Work out the finished part from the listing and answer in its coordinate system (mm). A direction names the side the tool comes from. Give positions to 0.01 mm unless a question says otherwise; leave off trailing zeros. Write each loop counter-clockwise with the first axis right and the second up, starting at its lowest first coordinate (ties: lowest second). Pieces come first, ordered by that corner, then holes.
1) Straight lines are drawn through the part: probe 1 along Y at (x, z) = (-7.55, 10); probe 2 along X at (y, z) = (3, 10.5); probe 3 along Y at (x, z) = (7, 10.5). For each, find the intervals that lie inside material, in ascending order.
2) Find section B-B (x = 0). Determine the outline of the cut face in (y, z) (3 decimals), plus the area to 3 significant figures.
3) Find section D-D (z = 6.75). Determine the outline of the cut face in (x, y).
4) Determine the mould class of faces 1 (the face through (7, 0, 0)), 2 (the face through (31, 9.76, 2.46)), 3 (the face through (25.543, -13.498, 2.524)) for opening direction X: pulls with the +X half, pulls with the -X half, needs draft (parallel to the pull), parting line crosses it, or undercut.
5) Find section A-A (z = 13). Determine the outline of the cut face in (x, y), plus the area to 3 significant figures.
6) A tool of negligible diameter and unlimited length cuts with its end or side. For faces 4 (the face through (10.503, 0, 11)), 5 (the face through (8, 10, 11)), 6 (the face through (-8, -6.2, 11.6)), 7 (the face through (8, -10, 11)), 8 (the face through (-11.26, 0.18, 5.71)), from which of +Z, -Z, +X, -X, +Y, -Y can it reach the whole face along a straight path? Write none if from no direction.
7) Given pin 1 Ø1.5 at (x, z) = (9, 10.5) entering from +Y; pin 2 Ø3 at (y, z) = (-1.5, 11) entering from +X; pin 3 Ø2.5 at (x, z) = (-8, 11) entering from -Y, each flat-ended and moving along its own axis, determine where each tip first touches the part or whether it passes through.
8) Find section C-C (y = -5). Determine the outline of the cut face in (x, z).
```python
from build123d import *

# Parameters (mm, degrees)
SKETCH_1_R                     = 32.5
EXTRUDE_1_DEPTH                = 5
PATTERN_CIRCULAR_1_COUNT       = 3
SKETCH_5_W                     = 5
SKETCH_5_H                     = 20
EXTRUDE_2_DEPTH                = 10
HOLE_WIZARD_M3_1_2_D           = 3.4
HOLE_WIZARD_M3_1_2_CBORE_D     = 6.5
HOLE_WIZARD_M3_1_2_CBORE_DEPTH = 3.4
F_4_0MM_1_D                    = 4
FILLET_1_R                     = 2.5
FILLET_2_R                     = 2.5


with BuildPart() as part:
    # 스케치1 → 보스-돌출1 (new body)
    with BuildSketch(Plane.XY):
        Circle(SKETCH_1_R)
    extrude(amount=EXTRUDE_1_DEPTH)

    # 스케치4 → Hole Wizard M3 _ _1 (revolve, cut)
    with BuildSketch(Plane(origin=(0, 27.5, 5), x_dir=(0, -1, 0), z_dir=(1, 0, 0))):
        Polygon((0, 0), (0, 6.021463052), (1.7, 5), (1.7, 0.020977491), (1.725, 0), align=None)
    hole_wizard_m3_1 = revolve(axis=Axis((0, 27.5, 11.35), (0, 0, -1)), mode=Mode.SUBTRACT)

    # 원형 패턴1: Hole Wizard M3 _ _1 ×3 about axis
    pattern_circular_1_axis = Axis((0, -0.077690761, 0), (0, 0, 1))
    for i in range(1, PATTERN_CIRCULAR_1_COUNT):
        add(hole_wizard_m3_1.rotate(pattern_circular_1_axis, i * 360 / PATTERN_CIRCULAR_1_COUNT), mode=Mode.SUBTRACT)

    # 스케치5 → 보스-돌출2 (add)
    with BuildSketch(Plane.XY.offset(5)):
        with Locations((-8.003327874, 0)):
            Rectangle(SKETCH_5_W, SKETCH_5_H)
        with Locations((8.003327874, 0)):
            Rectangle(SKETCH_5_W, SKETCH_5_H)
    extrude(amount=EXTRUDE_2_DEPTH)

    # Hole Wizard M3 _ _ _ _ _ _1 2 (through all)
    with Locations(Plane(origin=(0, 0, 0), x_dir=(-1, 0, 0), z_dir=(0, 0, -1))):
        with Locations((0, 0)):
            CounterBoreHole(HOLE_WIZARD_M3_1_2_D / 2, HOLE_WIZARD_M3_1_2_CBORE_D / 2, HOLE_WIZARD_M3_1_2_CBORE_DEPTH)

    # Ø4.0mm 맞춤핀 구멍1 (through all)
    with Locations(Plane.ZY.offset(10.503327874)):
        with Locations((10, 5), (10, -5)):
            Hole(F_4_0MM_1_D / 2)

    # 필렛1
    fillet_1_edges = [part.edges().sort_by_distance(p)[0] for p in [
        (-10.503327874, 0, 5),
        (10.503327874, 0, 5),
    ]]
    fillet(fillet_1_edges, radius=FILLET_1_R)

    # 필렛2
    fillet_2_edges = [part.edges().sort_by_distance(p)[0] for p in [
        (8.003327874, -10, 5),
        (-8.003327874, -10, 5),
        (8.003327874, 10, 5),
        (-8.003327874, 10, 5),
    ]]
    fillet(fillet_2_edges, radius=FILLET_2_R)


solid = part.part
```
Results:
1. probe 1: y = -10 to -7, -3 to 3, 7 to 10
1. probe 2: x = -10.5 to -5.5, 5.5 to 10.5
1. probe 3: y = -10 to -6.94, -3.06 to 3.06, 6.94 to 10
2. outline: (-32.5, 0) - (-3.25, 0) - (-3.25, 3.4) - (-1.7, 3.4) - (-1.7, 5) - (-32.5, 5) - close; (1.7, 3.4) - (3.25, 3.4) - (3.25, 0) - (25.8, 0) - (25.8, 4.979) - (25.775, 5) - (1.7, 5) - close; (29.2, 0) - (32.5, 0) - (32.5, 5) - (29.225, 5) - (29.2, 4.979) - close
2. area: 280 mm2
3. outline: (-10.62, -10.12) - (-5.5, -10.12) - (-5.5, 10.12) - (-10.62, 10.12) - close; (5.5, -10.12) - (10.62, -10.12) - (10.62, 10.12) - (5.5, 10.12) - close
4. face 1: needs draft
4. face 2: parting line crosses it
4. face 3: undercut
5. outline: (-10.5, -10) - (-5.5, -10) - (-5.5, 10) - (-10.5, 10) - close; (5.5, -10) - (10.5, -10) - (10.5, 10) - (5.5, 10) - close
5. area: 200 mm2
6. face 4: +Z, +X, +Y, -Y
6. face 5: +Z, +X, -X, +Y
6. face 6: +X, -X
6. face 7: +Z, +X, -X, -Y
6. face 8: +Z, -X, +Y, -Y
7. pin 1: stops at y = 10
7. pin 2: stops at x = 10.5
7. pin 3: stops at y = -10
8. outline: (-32.11, 0) - (32.11, 0) - (32.11, 5) - (13, 5) arc R2.5 cw to (10.5, 7.5) - (10.5, 8) - (5.5, 8) - (5.5, 5) - (-5.5, 5) - (-5.5, 8) - (-10.5, 8) - (-10.5, 7.5) arc R2.5 cw to (-13, 5) - (-32.11, 5) - close; (-10.5, 12) - (-5.5, 12) - (-5.5, 15) - (-10.5, 15) - close; (5.5, 12) - (10.5, 12) - (10.5, 15) - (5.5, 15) - close
